```python
from build123d import *

# Parameters (mm, degrees)
F0_W     = 1.5
F0_H     = 1.5
F1_DEPTH = 2
F2_W     = 1.5
F2_H     = 11.5
F3_DEPTH = 5
F4_W     = 8.5
F4_H     = 11.5
F5_DEPTH = 1.5
F6_R     = 2
F7_DEPTH = 25


with BuildPart() as f1:
    # F0 (on Top) → F1 (new body)
    with BuildSketch(Plane.XY):
        with Locations((8.05449, 7.874021)):
            Rectangle(F0_W, F0_H)
        with Locations((8.05449, 12.874021)):
            Rectangle(F0_W, F0_H)
        with Locations((8.05449, 17.874021)):
            Rectangle(F0_W, F0_H)
        with Locations((15.05449, 7.874021)):
            Rectangle(F0_W, F0_H)
        with Locations((15.05449, 12.874021)):
            Rectangle(F0_W, F0_H)
        with Locations((15.05449, 17.874021)):
            Rectangle(F0_W, F0_H)
    extrude(amount=F1_DEPTH)

    # F2 (on face) → F3 (join)
    with BuildSketch(Plane.XY.offset(2)):
        with Locations((8.05449, 12.874021)):
            Rectangle(F2_W, F2_H)
        with Locations((15.05449, 12.874021)):
            Rectangle(F2_W, F2_H)
    extrude(amount=F3_DEPTH)

    # F4 (on face) → F5 (join)
    with BuildSketch(Plane.XY.offset(7)):
        with Locations((11.55449, 12.874021)):
            Rectangle(F4_W, F4_H)
    extrude(amount=F5_DEPTH)

    # F6 (on face) → F7 (cut)
    with BuildSketch(Plane.XY.offset(8.5)):
        with Locations((11.55449, 12.874021)):
            Circle(F6_R)
    extrude(amount=-F7_DEPTH, mode=Mode.SUBTRACT)


solid = f1.part
```
Design review of the part built by this model. Coordinates are the model's own, in mm. A direction names the side the tool comes from. Give positions to 0.01 mm unless a question says otherwise; leave off trailing zeros. Write each loop counter-clockwise with the first axis right and the second up, starting at its lowest first coordinate (ties: lowest second). Pieces come first, ordered by that corner, then holes. Notation, with made-up numbers: (10.5, -4) -> (62.5, -4) arc R22 ccw to (62.5, 6) -> close; hole circle Ø11 at (5, 66.25). An arc over 180 degrees is marked (long way). Answer in a Markdown table with one row per item.
(1) Consider section C-C (x = 10). State the section outline as (y, z) points, then the cut area to 3 significant figures.
Results:
| item | result |
|---|---|
| outline | (7.12, 7) -> (11.62, 7) -> (11.62, 8.5) -> (7.12, 8.5) -> close; (14.13, 7) -> (18.62, 7) -> (18.62, 8.5) -> (14.13, 8.5) -> close |
| area | 13.5 mm2 |
(2) Consider section D-D (z = 1.75). State the section outline as (x, y) points.
Results:
| item | result |
|---|---|
| outline | (7.3, 7.12) -> (8.8, 7.12) -> (8.8, 8.62) -> (7.3, 8.62) -> close; (7.3, 12.12) -> (8.8, 12.12) -> (8.8, 13.62) -> (7.3, 13.62) -> close; (7.3, 17.12) -> (8.8, 17.12) -> (8.8, 18.62) -> (7.3, 18.62) -> close; (14.3, 7.12) -> (15.8, 7.12) -> (15.8, 8.62) -> (14.3, 8.62) -> close; (14.3, 12.12) -> (15.8, 12.12) -> (15.8, 13.62) -> (14.3, 13.62) -> close; (14.3, 17.12) -> (15.8, 17.12) -> (15.8, 18.62) -> (14.3, 18.62) -> close |
(3) Consider section A-A (z = 5.5). State the section outline as (x, y) points.
Results:
| item | result |
|---|---|
| outline | (7.3, 7.12) -> (8.8, 7.12) -> (8.8, 18.62) -> (7.3, 18.62) -> close; (14.3, 7.12) -> (15.8, 7.12) -> (15.8, 18.62) -> (14.3, 18.62) -> close |
(4) Consider section B-B (y = 12.5). State the section outline as (x, z) points, then the cut area to 3 significant figures.
Results:
| item | result |
|---|---|
| outline | (7.3, 0) -> (8.8, 0) -> (8.8, 7) -> (9.59, 7) -> (9.59, 8.5) -> (7.3, 8.5) -> close; (13.52, 7) -> (14.3, 7) -> (14.3, 0) -> (15.8, 0) -> (15.8, 8.5) -> (13.52, 8.5) -> close |
| area | 27.9 mm2 |
(5) Mouldability with a two-part tool opening along X and no side actions: class faces 1 (the flat face through (7.304, 13, 5)), 2 (the flat face through (14.304, 13, 4)), 3 (the flat face through (15, 18, 0)) as +X half, -X half, draft (parallel to the pull), parting line (faces both ways), or undercut.
Results:
| item | result |
|---|---|
| face 1 | -X half |
| face 2 | undercut |
| face 3 | draft |
(6) To check wall thickness, follow probe 1 along X at (y, z) = (11.25, 6.75); probe 2 along Z at (x, y) = (9.75, 9.5); probe 3 along Y at (x, z) = (10, 7.75). State the ranges of each line that lie inside material, in increasing order.
Results:
| item | result |
|---|---|
| probe 1 | 7.3 to 8.8, 14.3 to 15.8 |
| probe 2 | 7 to 8.5 |
| probe 3 | 7.12 to 11.62, 14.13 to 18.62 |
(7) For faces 4 (the flat face through (8, 10, 2)), 5 (the flat face through (13.35, 11.68, 7)), 6 (the flat face through (8, 13, 0)), list the 3-axis set-ups (+Z, -Z, +X, -X, +Y, -Y) from which the entire face can be reached by the end or side of a thin tool; tool diameter is ignored.
Results:
| item | result |
|---|---|
| face 4 | -Z, +X, -X |
| face 5 | -Z, +Y, -Y |
| face 6 | -Z, +X, -X, +Y, -Y |
(8) Clearance check with flat-ended pins moving along their axes: pin 1 (1.2 mm diameter, centred on x = 8, y = 10, fed in from -Z); pin 2 (1.5 mm diameter, centred on x = 10.5, y = 17, fed in from -Z). State where each tip first meets the part, or that it passes through.
Results:
| item | result |
|---|---|
| pin 1 | z = 2 |
| pin 2 | z = 7 |
